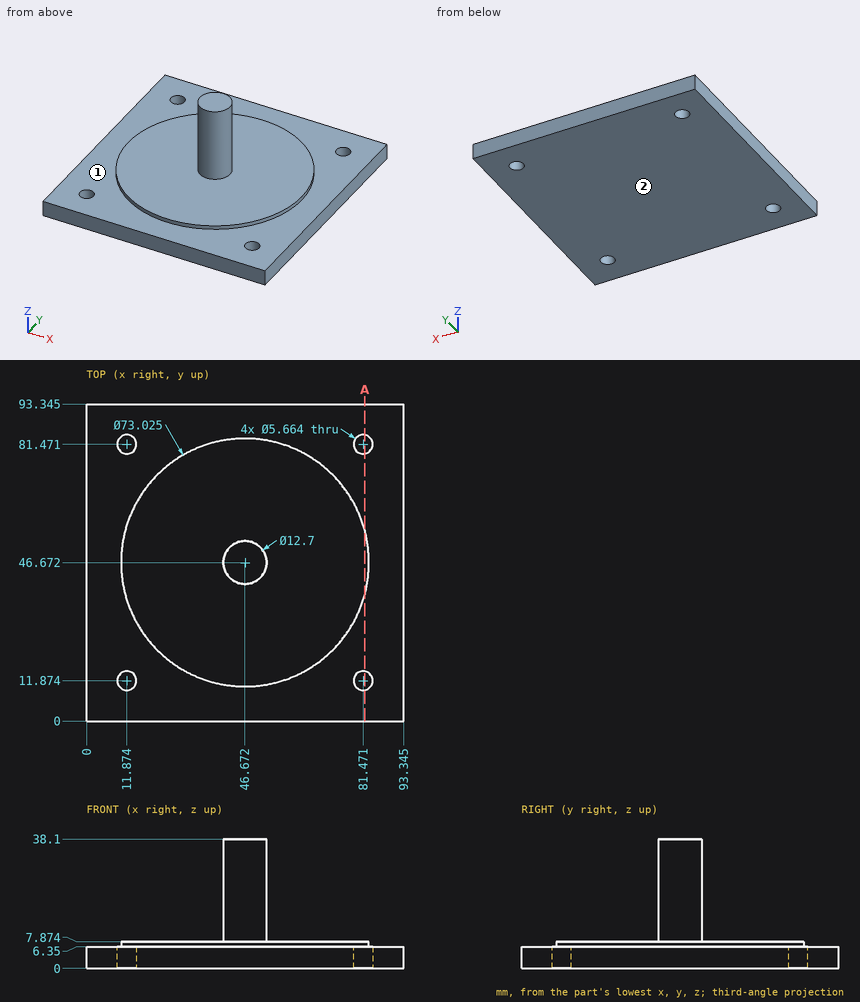
Input: dimensioned drawing with shaded views. Units: mm. Origin: part minimum x, y, z. A direction names the side the tool comes from. Round coordinates to 2 decimals unless told otherwise and drop trailing zeros. Answer as a JSON object with one key per item and string values. Group by question number.
Q1. Contact query for flat-ended pins moving along their axis: P1, Ø4.5, axis at x = 81.47, y = 81.47, coming from the +Z side; P2, Ø8, axis at y = 44, z = 11.5, coming from the -X side; P3, Ø7.5, axis at x = 81.47, y = 11.87, coming from the +Z side. Output: stop coordinate, or through.
Q2. Ray query, line 1 (Z direction, x = 52, y = 55) (1 decimal); line 2 (Z direction, x = 44, y = 89.5); line 3 (X direction, y = 50, z = 21) (1 decimal). Return the intervals inside material, ascending. Write a range as from..to.
Q3. Section query A-A (x = 82). State how many separate pieces and enclosed holes the cut face has, plus the area to 3 significant figures.
Q4. Access query for the marked faces 1 and 2. Directions: +Z, -Z, +X, -X, +Y, -Y. A direction counts if a zero-diameter tool reaches every point of the face in a straight line with its end or side. Return the directions, or none.
Completed:
{
 "1": {"P1": "through", "P2": "x = 10.17", "P3": "z = 6.35"},
 "2": {"line 1": "0..7.9", "line 2": "0..6.35", "line 3": "41.3..52.1"},
 "3": {"separate pieces": "3", "enclosed holes": "0", "area": "550 mm²"},
 "4": {"face 1": "+Z", "face 2": "-Z, +X, -X, +Y, -Y"}
}
